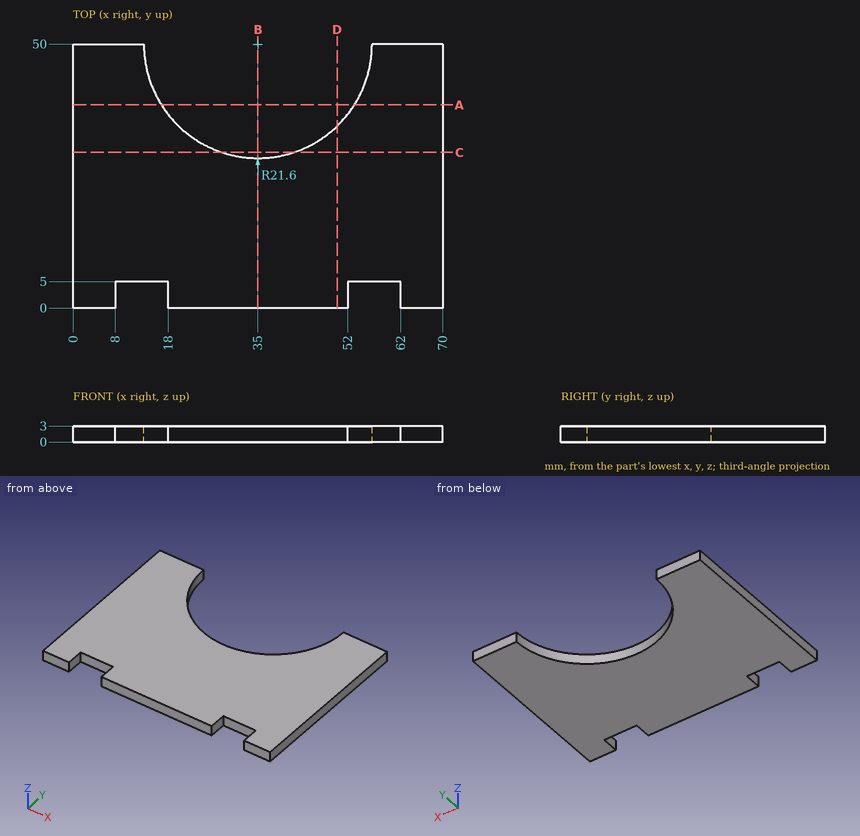
Verification items for this drawing (mm, ordinates from the low corner). Coordinates: 2 decimals unless noted, no trailing zeros. Order: outer loops, then holes, each group sorted by start corner. A loop starts at its lowest first (then second) coordinate and runs counter-clockwise, first axis right, second up. Notation, with made-up numbers: (39.5, 50) - (59.5, 50) arc R31 ccw to (59.5, 83) - close; hole circle Ø4 at (88.25, 5). An arc over 180 degrees is marked (long way). Answer as a JSON object with one key per item and string values. Group by question number.
Item 1: Sectioned sample at D-D, the plane x = 50. Record the cut outline in (y, z).
Item 2: Scan lines: probe 1 along Y at (x, z) = (57.5, 1.6); probe 2 along X at (y, z) = (32.5, 1.5); probe 3 along X at (y, z) = (34.5, 1.95). Record each from-to range of solid material in increasing order.
Item 3: Sectioned sample at B-B, the plane x = 35. Record the cut outline in (y, z), and give its area (3 significant figures).
Item 4: Sectioned sample at A-A, the plane y = 38.5. Record the cut outline in (x, z), and give its area (3 significant figures).
Item 5: Depth check by flat-ended pin: pin 1 Ø6 at (x, y) = (18.5, 34.5) entering from -Z; pin 2 Ø1.5 at (x, z) = (27, 2) entering from +Y; pin 3 Ø0.9 at (x, z) = (13.5, 2) entering from -Y. Enter the tip coordinate at first touch or a pass-through.
Item 6: Sectioned sample at C-C, the plane y = 29.5. Record the cut outline in (x, z), and give its area (3 significant figures).
Resolved:
{
 "1": {"outline": "(0, 0) - (34.46, 0) - (34.46, 3) - (0, 3) - close"},
 "2": {"probe 1": "5 to 50", "probe 2": "0 to 22.34, 47.66 to 70", "probe 3": "0 to 19.96, 50.04 to 70"},
 "3": {"outline": "(0, 0) - (28.4, 0) - (28.4, 3) - (0, 3) - close", "area": "85.2 mm^2"},
 "4": {"outline": "(0, 0) - (16.72, 0) - (16.72, 3) - (0, 3) - close; (53.28, 0) - (70, 0) - (70, 3) - (53.28, 3) - close", "area": "100 mm^2"},
 "5": {"pin 1": "z = 0", "pin 2": "y = 30.25", "pin 3": "y = 5"},
 "6": {"outline": "(0, 0) - (28.19, 0) - (28.19, 3) - (0, 3) - close; (41.81, 0) - (70, 0) - (70, 3) - (41.81, 3) - close", "area": "169 mm^2"}
}
